Part model, mm, in its own coordinate system. Face numbers are marked on the shaded views. A direction names the side the tool comes from. Give positions to 0.01 mm unless a question says otherwise; leave off trailing zeros. Order: outer loops, then holes, each group sorted by start corner. A loop starts at its lowest first (then second) coordinate and runs counter-clockwise, first axis right, second up. Notation, with made-up numbers: (3, 6) - (17, 6) arc R6 cw to (17, 17) - close; hole circle Ø8 at (-37.5, 29.5). An arc over 180 degrees is marked (long way). One line per item, written item: value.
```python
from build123d import *

# Parameters (mm, degrees)
SKETCH1_W           = 32
SKETCH1_H           = 6.5
BOSS_EXTRUDE1_DEPTH = 30
FILLET1_R           = 2
SKETCH2_R           = 4.1
CUT_EXTRUDE1_DEPTH  = 25.5
SKETCH3_R           = 4.1
CUT_EXTRUDE2_DEPTH  = 25.5
SKETCH5_W           = 32
SKETCH5_H           = 0.1
CUT_EXTRUDE3_DEPTH  = 37.629308734
SKETCH6_W           = 32
SKETCH6_H           = 1.8
CUT_EXTRUDE4_DEPTH  = 37.629308734
SKETCH7_R           = 2.2
CUT_EXTRUDE5_DEPTH  = 1.5
SKETCH8_R           = 1.2
CUT_EXTRUDE6_DEPTH  = 4
SKETCH9_R           = 1.2
CUT_EXTRUDE7_DEPTH  = 6
SKETCH10_R          = 2.2
CUT_EXTRUDE8_DEPTH  = 1.5
SKETCH11_R          = 1
CUT_EXTRUDE9_DEPTH  = 37.322647437
SKETCH12_R          = 1.7
CUT_EXTRUDE10_DEPTH = 1.5
SKETCH14_R          = 1.5
BOSS_EXTRUDE3_DEPTH = 11
SKETCH15_R          = 1.5
BOSS_EXTRUDE4_DEPTH = 11
FILLET2_R           = 2


with BuildPart() as part:
    # Sketch1 → Boss-Extrude1 (new body)
    with BuildSketch(Plane.XY):
        with Locations((3.954315745, -3.347843701)):
            Rectangle(SKETCH1_W, SKETCH1_H)
    extrude(amount=BOSS_EXTRUDE1_DEPTH)

    # Fillet1
    fillet1_edges = [part.edges().sort_by_distance(p)[0] for p in [
        (19.954315745, -3.347843701, 30),
        (-12.045684255, -3.347843701, 30),
        (19.954315745, -3.347843701, 0),
        (-12.045684255, -3.347843701, 0),
    ]]
    fillet(fillet1_edges, radius=FILLET1_R)

    # Sketch2 → Cut-Extrude1 (cut)
    with BuildSketch(Plane(origin=(0, 0, 0), x_dir=(-1, 0, 0), z_dir=(0, 0, -1))):
        with Locations((3.545684255, -0.197843701)):
            Circle(SKETCH2_R)
    extrude(amount=-CUT_EXTRUDE1_DEPTH, mode=Mode.SUBTRACT)

    # Sketch3 → Cut-Extrude2 (cut)
    with BuildSketch(Plane.XY.offset(30)):
        with Locations((11.454315745, -0.197843701)):
            Circle(SKETCH3_R)
    extrude(amount=-CUT_EXTRUDE2_DEPTH, mode=Mode.SUBTRACT)

    # Sketch5 → Cut-Extrude3 (cut, through all)
    with BuildSketch(Plane.XY.offset(30)):
        with Locations((3.954315745, -0.147843701)):
            Rectangle(SKETCH5_W, SKETCH5_H)
    extrude(amount=-CUT_EXTRUDE3_DEPTH, mode=Mode.SUBTRACT)

    # Sketch6 → Cut-Extrude4 (cut, through all)
    with BuildSketch(Plane.XY.offset(30)):
        with Locations((3.954315745, -5.697843701)):
            Rectangle(SKETCH6_W, SKETCH6_H)
    extrude(amount=-CUT_EXTRUDE4_DEPTH, mode=Mode.SUBTRACT)

    # Sketch7 → Cut-Extrude5 (cut)
    with BuildSketch(Plane.XZ.offset(4.797843701)):
        with Locations((-10.045684255, 2)):
            Circle(SKETCH7_R)
    extrude(amount=-CUT_EXTRUDE5_DEPTH, mode=Mode.SUBTRACT)

    # Sketch8 → Cut-Extrude6 (cut)
    with BuildSketch(Plane.XZ.offset(3.297843701)):
        with Locations((-10.045684255, 2)):
            Circle(SKETCH8_R)
    extrude(amount=-CUT_EXTRUDE6_DEPTH, mode=Mode.SUBTRACT)

    # Sketch9 → Cut-Extrude7 (cut)
    with BuildSketch(Plane.XZ.offset(4.797843701)):
        with Locations((-10.045684255, 28)):
            Circle(SKETCH9_R)
        with Locations((17.954315745, 28)):
            Circle(SKETCH9_R)
        with Locations((17.954315745, 2)):
            Circle(SKETCH9_R)
    extrude(amount=-CUT_EXTRUDE7_DEPTH, mode=Mode.SUBTRACT)

    # Sketch10 → Cut-Extrude8 (cut)
    with BuildSketch(Plane.XZ.offset(4.797843701)):
        with Locations((-10.045684255, 28)):
            Circle(SKETCH10_R)
        with Locations((17.954315745, 28)):
            Circle(SKETCH10_R)
        with Locations((17.954315745, 2)):
            Circle(SKETCH10_R)
    extrude(amount=-CUT_EXTRUDE8_DEPTH, mode=Mode.SUBTRACT)

    # Sketch11 → Cut-Extrude9 (cut, through all)
    with BuildSketch(Plane(origin=(0, -0.197843701, 0), x_dir=(1, 0, 0), z_dir=(0, 1, 0))):
        with Locations(Location((3.954315745, -3.6, 0), (0, 0, 270))):
            Circle(SKETCH11_R)
        with Locations(Location((3.954315745, -26.4, 0), (0, 0, 270))):
            Circle(SKETCH11_R)
    extrude(amount=-CUT_EXTRUDE9_DEPTH, mode=Mode.SUBTRACT)

    # Sketch12 → Cut-Extrude10 (cut)
    with BuildSketch(Plane.XZ.offset(4.797843701)):
        with Locations((3.954315745, 26.4)):
            Circle(SKETCH12_R)
        with Locations((3.954315745, 3.6)):
            Circle(SKETCH12_R)
    extrude(amount=-CUT_EXTRUDE10_DEPTH, mode=Mode.SUBTRACT)

    # Sketch14 → Boss-Extrude3 (add)
    with BuildSketch(Plane.XY.offset(4.5)):
        with Locations((11.454315745, -0.197843701)):
            Circle(SKETCH14_R)
    extrude(amount=-BOSS_EXTRUDE3_DEPTH)

    # Sketch15 → Boss-Extrude4 (add)
    with BuildSketch(Plane(origin=(0, 0, 25.5), x_dir=(-1, 0, 0), z_dir=(0, 0, -1))):
        with Locations((3.545684255, -0.197843701)):
            Circle(SKETCH15_R)
    extrude(amount=-BOSS_EXTRUDE4_DEPTH)

    # Fillet2
    # the kernel refuses this fillet: 2 mm, written as the material it takes off along each edge
    with BuildSketch(Plane(origin=(19.954315745, -4.797843701, 32.083484861), x_dir=(-1, 0, 0), z_dir=(0, 0, -1)), Plane(origin=(-12.045684255, -4.797843701, 32.083484861), x_dir=(0, 1, 0), z_dir=(0, 0, -1))) as fillet2_piece_1:
        with BuildLine():
            CenterArc((FILLET2_R, FILLET2_R), FILLET2_R, 180, 90)
            Line((0, FILLET2_R), (0, 0))
            Line((0, 0), (FILLET2_R, 0))
        make_face()
    extrude(amount=34.166969722, mode=Mode.SUBTRACT)


solid = part.part
```
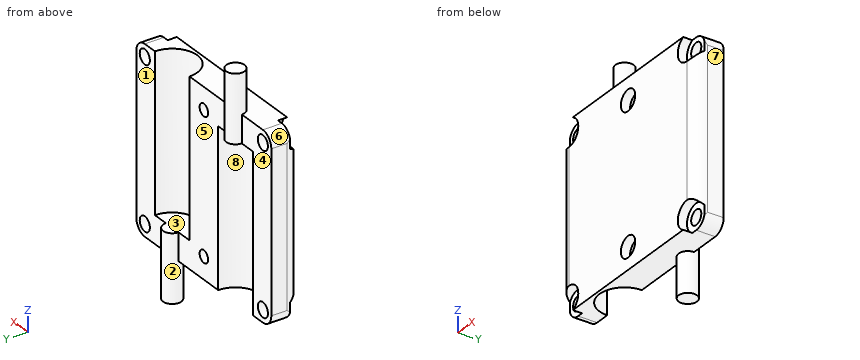
1) Slice it at A-A on x = 18.5. Write the cut outline in (y, z).
Answer:
outline: (-4.72, 4.13) - (-3.3, 4.13) - (-3.3, 3.07) - (-0.2, 3.07) - (-0.2, 26.93) - (-3.3, 26.93) - (-3.3, 25.87) - (-4.72, 25.87) - close; (-3.3, 0.08) - (-0.2, 0.08) - (-0.2, 0.93) - (-3.3, 0.93) - close; (-3.3, 29.07) - (-0.2, 29.07) - (-0.2, 29.92) - (-3.3, 29.92) - close
2) Which spindle directions (+Z, -Z, +X, -X, +Y, -Y) get a long thin tool onto all of the face, cutting with end or side? Do the marked faces 1, 2, 3 and 4. Say none if no direction does.
Answer:
face 1: +Z, -Z, +X, +Y
face 2: -Z
face 3: +Z, +Y
face 4: +Z, -Z, -X, +Y
3) Two-plate mould, pull along X, no slides. Class the marked faces 5, 6, 7 and 8: pulls with the +X half, pulls with the -X half, needs draft (parallel to the pull), parting line crosses it, or undercut.
Answer:
face 5: needs draft
face 6: pulls with the -X half
face 7: pulls with the +X half
face 8: undercut
4) Slice it at C-C on x = -1. Write the cut outline in (y, z).
Answer:
outline: (-4.8, 0) - (-3.41, 0) - (-3.41, 25.5) - (-0.2, 25.5) - (-0.2, 30) - (-4.8, 30) - close
5) Drop flat-ended pins along their axis: P1, Ø3, axis at x = 3.95, z = 3.6, coming from the -Y side; P2, Ø2, axis at y = -3, z = 5, coming from the -X side; P3, Ø1.9, axis at x = -10.05, z = 28, coming from the -Y side; P4, Ø4.5, axis at x = 3.95, z = 26.4, coming from the +Y side. Give the stop position or say it passes through.
Answer:
P1: stops at y = -3.3
P2: stops at x = -12.05
P3: passes through
P4: stops at y = -0.2
6) Wall check: line 1 along X through (y, z) = (-3.5, 25); line 2 along Z through (x, y) = (17, -2); line 3 along X through (y, z) = (-1.75, 5.5). Give the ranges that are in metal, low to high. Write a range as [from, to].
Answer:
line 1: x = [-11.92, -5.98], [-1.12, 2.99], [4.92, 9.02], [13.88, 19.83]
line 2: z = [0, 1.27], [2.73, 27.27], [28.73, 30]
line 3: x = [-12.05, -7.34], [0.25, 7.66], [15.25, 19.95]
7) Slice it at B-B on z = 32. Write the cut outline in (x, y).
Answer:
outline: circle Ø3 at (-3.55, -0.2)
